```python
from build123d import *

# Parameters (mm, degrees)
SKETCH1_W           = 80.1
SKETCH1_H           = 42
BOSS_EXTRUDE1_DEPTH = 6
SKETCH2_W           = 76.1
SKETCH2_H           = 38
CUT_EXTRUDE1_DEPTH  = 5.4
FILLET1_R           = 2


with BuildPart() as part:
    # Sketch1 → Boss-Extrude1 (new body)
    with BuildSketch(Plane.XY):
        with Locations((4.05, 0)):
            Rectangle(SKETCH1_W, SKETCH1_H)
    extrude(amount=BOSS_EXTRUDE1_DEPTH)

    # Sketch2 → Cut-Extrude1 (cut)
    with BuildSketch(Plane(origin=(0, 0, 0), x_dir=(-1, 0, 0), z_dir=(0, 0, -1))):
        with Locations((-4.05, 0)):
            Rectangle(SKETCH2_W, SKETCH2_H)
    extrude(amount=-CUT_EXTRUDE1_DEPTH, mode=Mode.SUBTRACT)

    # Fillet1
    fillet1_edges = [part.edges().sort_by_distance(p)[0] for p in [
        (-36, 21, 3),
        (44.1, 21, 3),
        (44.1, -21, 3),
        (-36, -21, 3),
    ]]
    fillet(fillet1_edges, radius=FILLET1_R)


solid = part.part
```
Input: part model. Units: mm. Frame: model coordinates. A direction names the side the tool comes from. Coordinates: 2 decimals unless noted, no trailing zeros. Loops run counter-clockwise (first coordinate to the right, second up) from the corner with the lowest first, then second, coordinate; pieces in that order, holes last.
Q1. Set-up query: faces 5 (the flat face through (5, 0, 5.4)), 6 (the flat face through (44.1, 0, 3)). Return all of +Z, -Z, +X, -X, +Y, -Y with unobstructed straight access to the full face (end or side cutting, diameter ignored); none if empty.
Results are:
face 5: -Z
face 6: +Z, -Z, +X, +Y, -Y
Q2. Mould query, pull axis Y, two halves, no side actions, for faces 1 (the flat face through (4, -21, 3)), 2 (the flat face through (42.1, 0, 3)), 3 (the flat face through (-36, 0, 3)), 4 (the cylindrical face through (43.5, 20.43, 3.04)). Classes: +Y half, -Y half, draft (parallel to the pull), parting line (faces both ways), or undercut.
Results are:
face 1: -Y half
face 2: undercut
face 3: draft
face 4: +Y half
Q3. Section C-C, the plane y = -14. Return the cut outline in (x, z).
Results are:
outline: (-36, 0) - (-34, 0) - (-34, 5.4) - (42.1, 5.4) - (42.1, 0) - (44.1, 0) - (44.1, 6) - (-36, 6) - close
Q4. Section A-A, the plane x = 12.5. Return the cut outline in (y, z).
Results are:
outline: (-21, 0) - (-19, 0) - (-19, 5.4) - (19, 5.4) - (19, 0) - (21, 0) - (21, 6) - (-21, 6) - close
Q5. Section B-B, the plane z = 4.6. Return the cut outline in (x, y), and give its area (3 significant figures).
Results are:
outline: (-36, -19) arc R2 ccw to (-34, -21) - (42.1, -21) arc R2 ccw to (44.1, -19) - (44.1, 19) arc R2 ccw to (42.1, 21) - (-34, 21) arc R2 ccw to (-36, 19) - close; hole (-34, -19) - (42.1, -19) - (42.1, 19) - (-34, 19) - close
area: 469 mm2
Q6. Line query: line 1 along Y through (x, z) = (27.5, 4.65); line 2 along X through (y, z) = (-1, 0.35); line 3 along Z through (x, y) = (23.5, -4). Output: solid intervals per line, ascending.
Results are:
line 1: y = -21 to -19, 19 to 21
line 2: x = -36 to -34, 42.1 to 44.1
line 3: z = 5.4 to 6
Q7. Contact query for a flat-ended pin moving along its axis: pin 1 (1 mm diameter, centred on x = 11, y = -6, fed in from -Z). Output: stop coordinate, or through.
Results are:
pin 1: stops at z = 5.4
